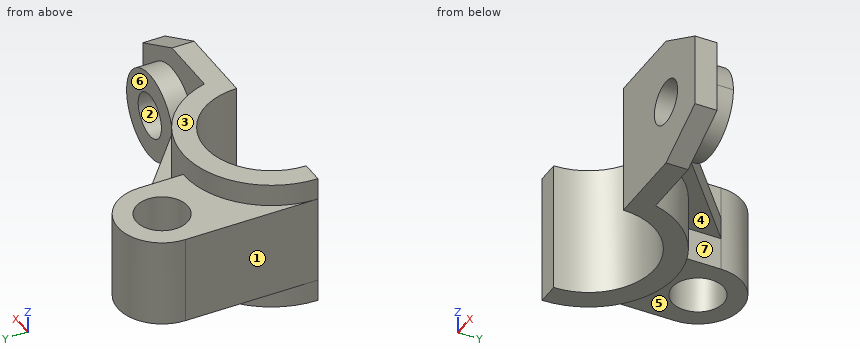
```python
from build123d import *
from build123d.topology import SkipClean

# Parameters (mm, degrees)
BOSS_EXTRUDE1_DEPTH        = 18
SKETCH1_3_R                = 12
SKETCH1_3_R_2              = 7
BOSS_EXTRUDE2_DEPTH        = 12
SKETCH2_R                  = 12
BOSS_EXTRUDE3_DEPTH        = 6
RIB1_REACH                 = 77.186
SKETCH3_WALL_W             = 189.251047722
SKETCH3_WALL_H             = 6
CHAMFER1_SIZE              = 8
CHAMFER1_SIZE2             = 15
CHAMFER2_SIZE              = 15
CHAMFER2_SIZE2             = 8
F_12_0MM_DOWEL_HOLE1_D     = 12
F_12_0MM_DOWEL_HOLE1_DEPTH = 30
F_12_0MM_DOWEL_HOLE1_TIP   = 3.605163714


with BuildPart() as part:
    # Sketch1 → Boss-Extrude1 (new, symmetric)
    with BuildSketch(Plane.XY):
        with BuildLine():
            ThreePointArc((18, 0), (0, 18), (-18, 0))
            Line((-18, 0), (-24, 0))
            ThreePointArc((-24, 0), (-3.02410302, 23.80871271), (23.237900077, 6))
            Line((23.237900077, 6), (55, 6))
            Line((55, 6), (55, 0))
            Line((55, 0), (24, 0))
            Line((24, 0), (18, 0))
        make_face()
    extrude(amount=BOSS_EXTRUDE1_DEPTH, both=True)

    # Sketch1<3> → Boss-Extrude2 (add, symmetric)
    # profile 1 of 2: a face of its own
    with BuildSketch(Plane.XY):
        with BuildLine():
            Line((-24, 36), (-24, 0))
            ThreePointArc((-24, 0), (-16.970562748, 16.970562748), (0, 24))
            Line((0, 24), (0, 36))
            ThreePointArc((0, 36), (-12, 24), (-24, 36))
        make_face()
    # profile 2 of 2: a face of its own
    with BuildSketch(Plane.XY):
        with Locations((-12, 36)):
            Circle(SKETCH1_3_R)
        with Locations((-12, 36)):
            Circle(SKETCH1_3_R_2, mode=Mode.SUBTRACT)
    extrude(amount=BOSS_EXTRUDE2_DEPTH, both=True)

    # Sketch2 → Boss-Extrude3 (add)
    with SkipClean():  # the faces are left unmerged after this step: merging them gives an invalid solid
        with BuildSketch(Plane(origin=(0, 6, 0), x_dir=(1, 0, 0), z_dir=(0, 1, 0))):
            with Locations((40, 0)):
                Circle(SKETCH2_R)
        extrude(amount=BOSS_EXTRUDE3_DEPTH)
    add(part.part.scale(1), mode=Mode.REPLACE)  # the faces are merged on a copy

    # Sketch3 wall → Rib1 (add, up to next)
    with BuildSketch(Plane(origin=(14, 24, 0), x_dir=(0.759256602365, -0.650791373456, 0), z_dir=(0.650791373456, 0.759256602365, 0)), mode=Mode.PRIVATE) as rib1_sk1:
        Rectangle(SKETCH3_WALL_W, SKETCH3_WALL_H)
    rib1_tool1 = extrude(rib1_sk1.sketch, amount=-RIB1_REACH, mode=Mode.PRIVATE) - part.part
    add(rib1_tool1.solids().sort_by_distance((14, 24, 0))[0])

    # Chamfer1
    chamfer1_edges = [part.edges().sort_by_distance(p)[0] for p in [
        (55, 3, 18),
    ]]
    chamfer1_side = [part.faces().sort_by_distance(p)[0] for p in [
        (55, 3, 0),
    ]]
    chamfer(chamfer1_edges, length=CHAMFER1_SIZE, length2=CHAMFER1_SIZE2, reference=chamfer1_side[0])

    # Chamfer2
    chamfer2_edges = [part.edges().sort_by_distance(p)[0] for p in [
        (55, 3, -18),
    ]]
    chamfer2_side = [part.faces().sort_by_distance(p)[0] for p in [
        (39.118950039, 5.174348742, -18),
    ]]
    chamfer(chamfer2_edges, length=CHAMFER2_SIZE, length2=CHAMFER2_SIZE2, reference=chamfer2_side[0])

    # Ø12.0mm Dowel Hole1
    with Locations(Plane(origin=(40, 12, 0), x_dir=(1, 0, 0), z_dir=(0, 1, 0))):
        with Locations((0, 0)):
            Hole(F_12_0MM_DOWEL_HOLE1_D / 2, depth=F_12_0MM_DOWEL_HOLE1_DEPTH)
            with Locations((0, 0, -(F_12_0MM_DOWEL_HOLE1_DEPTH + F_12_0MM_DOWEL_HOLE1_TIP / 2))):  # 118° drill point
                Cone(0, F_12_0MM_DOWEL_HOLE1_D / 2, F_12_0MM_DOWEL_HOLE1_TIP, mode=Mode.SUBTRACT)


solid = part.part
```
Work out the finished part from the listing and answer in its coordinate system (mm). Face numbers are marked on the shaded views. A direction names the side the tool comes from. Coordinates: 2 decimals unless noted, no trailing zeros. Write each loop counter-clockwise with the first axis right and the second up, starting at its lowest first coordinate (ties: lowest second). Pieces come first, ordered by that corner, then holes.
Q1. A cutting plane is placed at B-B, the plane x = -12. Give the vertices of the cut face in (y, z), then the cut area to 3 significant figures.
Q2. Find the intervals of material crossed by line 1 (Z direction, x = 40, y = 6.75); line 2 (X direction, y = 6.5, z = -0.5); line 3 (Z direction, x = -4.5, y = 24), in increasing order.
Q3. Which of the six approach directions +Z, -Z, +X, -X, +Y, -Y give full straight-line access (tool end or side, diameter ignored) to the marked faces 4, 5, 6 and 7?
Q4. Each of these flat-tipped pins is pushed along its axis until it touches: pin 1 Ø2.5 at (y, z) = (29, -6.5) entering from +X; pin 2 Ø9.5 at (x, z) = (45, 3) entering from +Y; pin 3 Ø11 at (x, z) = (40, 0) entering from +Y; pin 4 Ø16 at (x, y) = (-12, 36) entering from -Z. Where does it stop, or does it pass through?
Q5. A cutting plane is placed at D-D, the plane z = 14. Give the vertices of the cut face in (x, y), then the cut area to 3 significant figures.
Q6. Determine the mould class of the marked faces 1, 2 and 3 for opening direction Z: released by +Z, released by -Z, zero draft, split by the parting line, or undercut.
Q7. A cutting plane is placed at A-A, the plane y = 4.5. Give the vertices of the cut face in (x, z), then the cut area to 3 significant figures.
Q8. A cutting plane is placed at C-C, the plane y = 38. Give the vertices of the cut face in (x, z), then the cut area to 3 significant figures.
Findings below:
1. outline: (13.42, -18) - (20.78, -18) - (20.78, -12) - (29, -12) - (29, 12) - (20.78, 12) - (20.78, 18) - (13.42, 18) - close; (43, -12) - (48, -12) - (48, 12) - (43, 12) - close
1. area: 582 mm2
2. line 1: z = -12 to -6, 6 to 12
2. line 2: x = -24 to -16.79, 16.79 to 34.02, 45.98 to 51.99
2. line 3: z = -12 to 12
3. face 4: -Z, +Y
3. face 5: -Z, -X, +Y
3. face 6: +Z, -Z, +X, +Y
3. face 7: -Z, +X, +Y
4. pin 1: stops at x = 0
4. pin 2: stops at y = 12
4. pin 3: passes through
4. pin 4: stops at z = -12
5. outline: (-24, 0) - (-18, 0) arc R18 cw to (18, 0) - (47.5, 0) - (47.5, 6) - (23.24, 6) arc R24 ccw to start
5. area: 538 mm2
6. face 1: zero draft
6. face 2: undercut
6. face 3: released by +Z
7. outline: (-24, -12) - (-23.57, -12) - (-23.57, -18) - (-17.43, -18) - (-17.43, 18) - (-23.57, 18) - (-23.57, 12) - (-24, 12) - close; (17.43, -18) - (40, -18) - (55, -10) - (55, 10) - (40, 18) - (17.43, 18) - close; hole circle Ø12 at (40, 0)
7. area: 1,350 mm2
8. outline: (-23.83, -12) - (-18.71, -12) - (-18.71, 12) - (-23.83, 12) - close; (-5.29, -12) - (-0.17, -12) - (-0.17, 12) - (-5.29, 12) - close
8. area: 246 mm2
